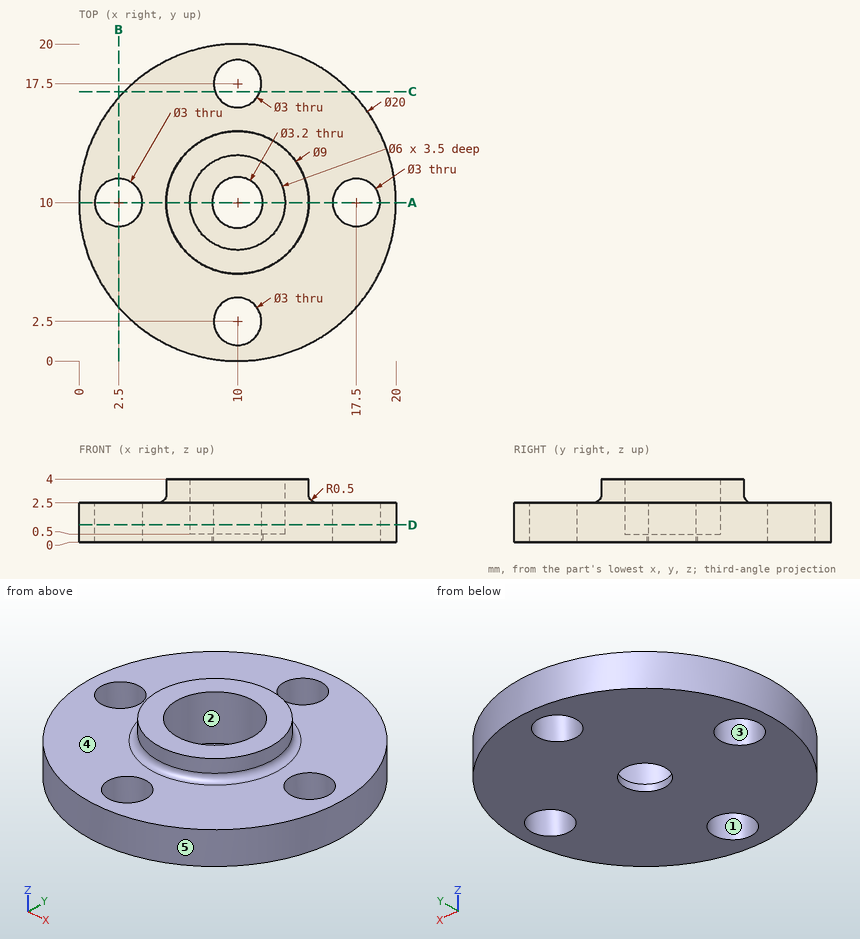
Part print with two shaded views. Sizes in mm from the minimum x, y, z corner. A direction names the side the tool comes from. Coordinates: 2 decimals unless noted, no trailing zeros. Write each loop counter-clockwise with the first axis right and the second up, starting at its lowest first coordinate (ties: lowest second). Pieces come first, ordered by that corner, then holes. Notation, with made-up numbers: (-25, -21.5) - (20, -21.5) arc R32 ccw to (20, 11.5) - close; hole circle Ø10 at (1, 13.25). An arc over 180 degrees is marked (long way). Put each result on its own line as item: value.
1. Probe line 1 along Y through (x, z) = (10, 1.85); line 2 along X through (y, z) = (8.25, 1.75); line 3 along Y through (x, z) = (12.75, 2.65). List the from-to ranges inside material, lowest first. Write a range as [from, to].
Final values:
line 1: y = [0, 1], [4, 7], [13, 16], [19, 20]
line 2: x = [0.15, 7.56], [12.44, 19.85]
line 3: y = [6.26, 8.8], [11.2, 13.74]
2. Band-saw the part on A-A (y = 10). Write the cut outline in (x, z).
Final values:
outline: (0, 0) - (1, 0) - (1, 2.5) - (0, 2.5) - close; (4, 0) - (8.4, 0) - (8.4, 0.5) - (7, 0.5) - (7, 4) - (5.5, 4) - (5.5, 3) arc R0.5 cw to (5, 2.5) - (4, 2.5) - close; (11.6, 0) - (16, 0) - (16, 2.5) - (15, 2.5) arc R0.5 cw to (14.5, 3) - (14.5, 4) - (13, 4) - (13, 0.5) - (11.6, 0.5) - close; (19, 0) - (20, 0) - (20, 2.5) - (19, 2.5) - close
3. Band-saw the part on B-B (x = 2.5). Write the cut outline in (y, z).
Final values:
outline: (3.39, 0) - (8.5, 0) - (8.5, 2.5) - (3.39, 2.5) - close; (11.5, 0) - (16.61, 0) - (16.61, 2.5) - (11.5, 2.5) - close
4. 3-axis set-ups, long thin cutter, end or side, ignore diameter. For the marked faces 1 and 2: which of +Z, -Z, +X, -X, +Y, -Y reach the whole face in a straight line?
Final values:
face 1: +Z, -Z
face 2: +Z
5. Two-plate mould, pull along X, no slides. Class the marked faces 3, 4 and 5: +X half, -X half, draft (parallel to the pull), parting line (faces both ways), or undercut.
Final values:
face 3: undercut
face 4: draft
face 5: parting line
6. Flat gauge pins, fed straight in: pin 1 Ø1.5 at (x, z) = (5.5, 1.5) entering from +Y; pin 2 Ø1.8 at (x, y) = (10.5, 11) entering from +Z; pin 3 Ø1.5 at (x, z) = (18, 1) entering from +Y. Where does each tip first touch, or does it go through?
Final values:
pin 1: stops at y = 19.27
pin 2: stops at z = 0.5
pin 3: stops at y = 16.89
7. Band-saw the part on D-D (z = 1.1). Write the cut outline in (x, y).
Final values:
outline: circle Ø20 at (10, 10); hole circle Ø3 at (2.5, 10); hole circle Ø6 at (10, 10); hole circle Ø3 at (10, 2.5); hole circle Ø3 at (10, 17.5); hole circle Ø3 at (17.5, 10)
8. Band-saw the part on C-C (y = 17). Write the cut outline in (x, z).
Final values:
outline: (2.86, 0) - (8.59, 0) - (8.59, 2.5) - (2.86, 2.5) - close; (11.41, 0) - (17.14, 0) - (17.14, 2.5) - (11.41, 2.5) - close
